Here's how the part is built. I have some questions about the finished solid (model axes, mm). Round coordinates to 2 decimals unless told otherwise and drop trailing zeros. Put each result on its own line as item: value. Start each with the question number.
1) I want a section at A-A, the plane z = 201. Give the number of separate pieces and of enclosed holes in the cut face, then the cut area to 3 significant figures.
2) Will these pins go through, and if not, where does the flat tip stop? P1, Ø1, axis at x = 25, y = 0.5, coming from the -Z side; P2, Ø1.4, axis at x = -1, z = 126.5, coming from the +Y side; P3, Ø3, axis at x = 1.5, z = 290.5, coming from the -Y side; P4, Ø3, axis at y = 2, z = 206.5, coming from the -X side.
3) If I drill on line 1 along X through (y, z) = (8, 468.5); line 2 along Y through (x, z) = (0, 202.5) (3 decimals); line 3 along Y through (x, z) = (11.5, 467), over which ranges is the centre line in solid material (lowest first)? Write a range as [from, to].
from build123d import *

# Parameters (mm, degrees)
SKETCH_R  = 2.1
PAD_DEPTH = 500


with BuildPart() as part:
    # Sketch → Pad (new body)
    with BuildSketch(Plane.XY):
        with BuildLine():
            Line((-10, 4.58), (-10, 9.5))
            ThreePointArc((-9.5, 10), (-9.853553, 9.853553), (-10, 9.5))
            Line((-9.5, 10), (-4.58, 10))
            Line((-4.58, 10), (-3.125, 8.545))
            Line((-3.125, 8.545), (-3.125, 8.2))
            Line((-5.5, 8.2), (-3.125, 8.2))
            Line((-5.5, 8.2), (-5.5, 6.56066))
            Line((-5.5, 6.56066), (-2.83934, 3.9))
            Line((-0.125, 3.9), (-2.83934, 3.9))
            ThreePointArc((-0.125, 3.9), (0, 3.775), (0.125, 3.9))
            Line((0.125, 3.9), (2.83934, 3.9))
            Line((2.83934, 3.9), (5.5, 6.56066))
            Line((5.5, 6.56066), (5.5, 8.2))
            Line((5.5, 8.2), (3.125, 8.2))
            Line((3.125, 8.2), (3.125, 8.545))
            Line((3.125, 8.545), (4.58, 10))
            Line((4.58, 10), (15.42, 10))
            Line((15.42, 10), (16.875, 8.545))
            Line((16.875, 8.545), (16.875, 8.2))
            Line((16.875, 8.2), (14.5, 8.2))
            Line((14.5, 8.2), (14.5, 6.56066))
            Line((14.5, 6.56066), (17.16066, 3.9))
            Line((17.16066, 3.9), (19.875, 3.9))
            ThreePointArc((19.875, 3.9), (20, 3.775), (20.125, 3.9))
            Line((20.125, 3.9), (22.83934, 3.9))
            Line((22.83934, 3.9), (25.5, 6.56066))
            Line((25.5, 6.56066), (25.5, 8.2))
            Line((25.5, 8.2), (23.125, 8.2))
            Line((23.125, 8.2), (23.125, 8.545))
            Line((23.125, 8.545), (24.58, 10))
            Line((24.58, 10), (29.5, 10))
            ThreePointArc((30, 9.5), (29.853554, 9.853554), (29.5, 10))
            Line((30, 9.5), (30, 4.58))
            Line((30, 4.58), (28.545, 3.125))
            Line((28.545, 3.125), (28.2, 3.125))
            Line((28.2, 3.125), (28.2, 5.5))
            Line((28.2, 5.5), (26.560661, 5.5))
            Line((26.560661, 5.5), (23.9, 2.83934))
            Line((23.9, 2.83934), (23.9, 0.125))
            ThreePointArc((23.9, 0.125), (23.775, 2e-06), (23.899997, -0.125))
            Line((23.899997, -2.83934), (23.899997, -0.125))
            Line((26.560658, -5.5), (23.899997, -2.83934))
            Line((28.199997, -5.5), (26.560658, -5.5))
            Line((28.199997, -3.125), (28.199997, -5.5))
            Line((28.544997, -3.125), (28.199997, -3.125))
            Line((29.999997, -4.58), (28.544997, -3.125))
            Line((29.999997, -9.5), (29.999997, -4.58))
            ThreePointArc((29.5, -10), (29.853552, -9.853552), (29.999997, -9.5))
            Line((24.58, -10), (29.5, -10))
            Line((23.125, -8.545), (24.58, -10))
            Line((23.125, -8.2), (23.125, -8.545))
            Line((25.5, -8.2), (23.125, -8.2))
            Line((25.5, -6.56066), (25.5, -8.2))
            Line((22.83934, -3.9), (25.5, -6.56066))
            Line((20.125, -3.9), (22.83934, -3.9))
            ThreePointArc((20.125, -3.9), (20, -3.775), (19.875, -3.9))
            Line((17.16066, -3.9), (19.875, -3.9))
            Line((14.5, -6.56066), (17.16066, -3.9))
            Line((14.5, -8.2), (14.5, -6.56066))
            Line((16.875, -8.2), (14.5, -8.2))
            Line((16.875, -8.545), (16.875, -8.2))
            Line((15.42, -10), (16.875, -8.545))
            Line((4.58, -10), (15.42, -10))
            Line((4.58, -10), (3.125, -8.545))
            Line((3.125, -8.545), (3.125, -8.2))
            Line((3.125, -8.2), (5.5, -8.2))
            Line((5.5, -8.2), (5.5, -6.56066))
            Line((2.83934, -3.9), (5.5, -6.56066))
            Line((0.125, -3.9), (2.83934, -3.9))
            ThreePointArc((0.125, -3.9), (0, -3.775), (-0.125, -3.9))
            Line((-0.125, -3.9), (-2.83934, -3.9))
            Line((-2.83934, -3.9), (-5.5, -6.56066))
            Line((-5.5, -6.56066), (-5.5, -8.2))
            Line((-5.5, -8.2), (-3.125, -8.2))
            Line((-3.125, -8.545), (-3.125, -8.2))
            Line((-4.58, -10), (-3.125, -8.545))
            Line((-9.5, -10), (-4.58, -10))
            ThreePointArc((-10, -9.5), (-9.853553, -9.853553), (-9.5, -10))
            Line((-10, -4.58), (-10, -9.5))
            Line((-8.545, -3.125), (-10, -4.58))
            Line((-8.2, -3.125), (-8.545, -3.125))
            Line((-8.2, -5.5), (-8.2, -3.125))
            Line((-6.56066, -5.5), (-8.2, -5.5))
            Line((-3.9, -2.83934), (-6.56066, -5.5))
            Line((-3.9, -0.125), (-3.9, -2.83934))
            ThreePointArc((-3.9, -0.125), (-3.775, 0), (-3.9, 0.125))
            Line((-3.9, 2.83934), (-3.9, 0.125))
            Line((-6.56066, 5.5), (-3.9, 2.83934))
            Line((-8.2, 5.5), (-6.56066, 5.5))
            Line((-8.2, 5.5), (-8.2, 3.125))
            Line((-8.545, 3.125), (-8.2, 3.125))
            Line((-10, 4.58), (-8.545, 3.125))
        make_face()
        Circle(SKETCH_R, mode=Mode.SUBTRACT)
        with Locations((20, 0)):
            Circle(SKETCH_R, mode=Mode.SUBTRACT)
        with BuildLine():
            Line((7, 5.93934), (3.9, 2.83934))
            Line((3.9, 2.83934), (3.9, 0.125))
            ThreePointArc((3.9, 0.125), (3.775, 0), (3.9, -0.125))
            Line((3.9, -0.125), (3.9, -2.83934))
            Line((3.9, -2.83934), (7, -5.93934))
            Line((7, -5.93934), (7, -8.2))
            Line((7, -8.2), (13, -8.2))
            Line((13, -8.2), (13, -5.93934))
            Line((13, -5.93934), (16.1, -2.83934))
            Line((16.1, -2.83934), (16.1, -0.125))
            ThreePointArc((16.1, -0.125), (16.224999, 0), (16.1, 0.125))
            Line((16.1, 2.83934), (16.1, 0.125))
            Line((13, 5.93934), (16.1, 2.83934))
            Line((13, 8.2), (13, 5.93934))
            Line((7, 8.2), (13, 8.2))
            Line((7, 5.93934), (7, 8.2))
        make_face(mode=Mode.SUBTRACT)
    extrude(amount=PAD_DEPTH)


solid = part.part
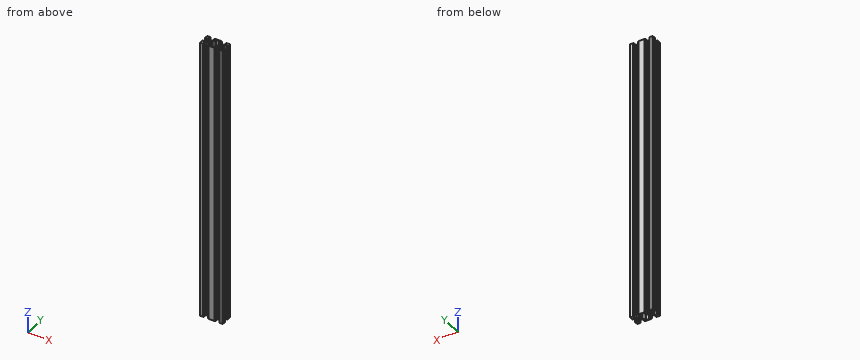
Findings:
1. separate pieces: 1
1. enclosed holes: 3
1. area: 298 mm2
2. P1: passes through
2. P2: stops at y = 3.9
2. P3: stops at y = -4.06
2. P4: stops at x = -8.92
3. line 1: x = [-10, -5.5], [5.5, 7], [13, 14.5], [25.5, 30]
3. line 2: y = [-3.775, -2.1], [2.1, 3.775]
3. line 3: y = [-10, -8.2], [8.2, 10]
